```python
from build123d import *

# Parameters (mm, degrees)
BOSS_EXTRUDE1_DEPTH = 48.26
SKETCH2_W           = 9.525
SKETCH2_H           = 22.352
CUT_EXTRUDE1_DEPTH  = 56.99533552
SKETCH3_R           = 1.2192
CUT_EXTRUDE2_DEPTH  = 56.99533552
FILLET2_R           = 1.5875
SKETCH4_R           = 2.5527
CUT_EXTRUDE3_DEPTH  = 56.995335629
CUT_EXTRUDE4_DEPTH  = 56.995335629
CHAMFER2_SIZE       = 6.35
CHAMFER2_SIZE2      = 10.998522628


with BuildPart() as part:
    # Sketch1 → Boss-Extrude1 (new body)
    with BuildSketch(Plane.XY):
        with BuildLine():
            Line((0, 0), (0, -25.4))
            Line((0, -25.4), (1.5875, -25.4))
            ThreePointArc((1.5875, -25.4), (2.710032015, -24.935032015), (3.175, -23.8125))
            Line((3.175, -23.8125), (3.175, -4.7625))
            ThreePointArc((3.175, -4.7625), (3.639967985, -3.639967985), (4.7625, -3.175))
            Line((4.7625, -3.175), (11.1125, -3.175))
            ThreePointArc((11.1125, -3.175), (12.235032015, -2.710032015), (12.7, -1.5875))
            Line((12.7, -1.5875), (12.7, 0))
            Line((12.7, 0), (0, 0))
        make_face()
    extrude(amount=BOSS_EXTRUDE1_DEPTH)

    # Sketch2 → Cut-Extrude1 (cut, through all)
    with BuildSketch(Plane(origin=(0, 0, 0), x_dir=(0, 0, -1), z_dir=(1, 0, 0))):
        with Locations((-4.7625, -14.224)):
            Rectangle(SKETCH2_W, SKETCH2_H)
    extrude(amount=CUT_EXTRUDE1_DEPTH, mode=Mode.SUBTRACT)

    # Sketch3 → Cut-Extrude2 (cut, through all)
    with BuildSketch(Plane(origin=(0, 0, 0), x_dir=(1, 0, 0), z_dir=(0, 1, 0))):
        with Locations(Location((2.794, -3.175, 0), (0, 0, 180))):
            Circle(SKETCH3_R)
        with Locations(Location((7.874, -3.175, 0), (0, 0, 180))):
            Circle(SKETCH3_R)
    extrude(amount=-CUT_EXTRUDE2_DEPTH, mode=Mode.SUBTRACT)

    # Fillet2
    fillet2_edges = [part.edges().sort_by_distance(p)[0] for p in [
        (5.867335197, -3.048, 9.525),
    ]]
    fillet(fillet2_edges, radius=FILLET2_R)

    # Sketch4 → Cut-Extrude3 (cut, through all)
    with BuildSketch(Plane.ZY):
        with Locations(Location((25.4, -9.398, 0), (0, 0, 270))):
            Circle(SKETCH4_R)
    extrude(amount=-CUT_EXTRUDE3_DEPTH, mode=Mode.SUBTRACT)

    # Sketch6 → Cut-Extrude4 (cut, through all)
    with BuildSketch(Plane(origin=(0, 0, 0), x_dir=(1, 0, 0), z_dir=(0, 1, 0))):
        Polygon((5.08, -48.26), (12.7, -1.5875), (12.7, -48.26), align=None)
    extrude(amount=-CUT_EXTRUDE4_DEPTH, mode=Mode.SUBTRACT)

    # Chamfer2
    chamfer2_edges = [part.edges().sort_by_distance(p)[0] for p in [
        (2.54, 0, 48.26),
    ]]
    chamfer2_side = [part.faces().sort_by_distance(p)[0] for p in [
        (1.769133551, -11.790484545, 48.26),
    ]]
    chamfer(chamfer2_edges, length=CHAMFER2_SIZE, length2=CHAMFER2_SIZE2, reference=chamfer2_side[0])


solid = part.part
```
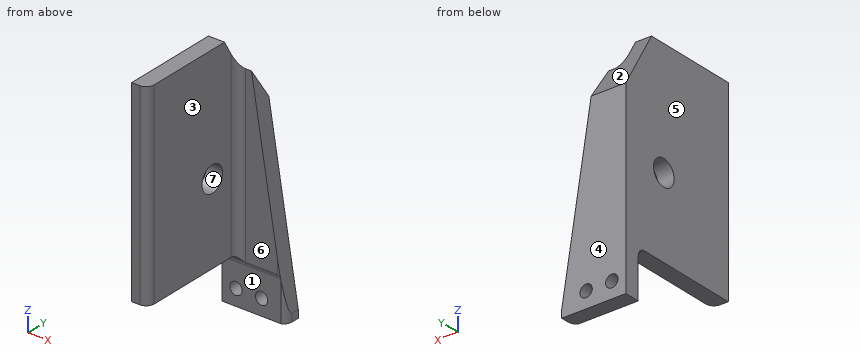
Geometry check sheet. Reference: the model listing, model coordinates, mm. Face numbers are marked on the shaded views. A direction names the side the tool comes from. Give positions to 0.01 mm unless a question says otherwise; leave off trailing zeros. Order: outer loops, then holes, each group sorted by start corner. A loop starts at its lowest first (then second) coordinate and runs counter-clockwise, first axis right, second up.
1. Access from +Z, -Z, +X, -X, +Y, -Y to the whole of each face (thin tool, end or side, straight path). Record for the marked faces 1, 2 and 3.
2. Thickness scan on L1, parallel to X at y = -1.5, z = 4; L2, parallel to X at y = -9, z = 39 (3 decimals); L3, parallel to Y at x = 2.5, z = 25.5. Record the ranges inside material, lowest first.
3. Section check C-C, the plane y = -2.25. Enter the section's corners in (x, z) (3 decimals), and give its area (3 significant figures).
4. Gauge pin test, flat ends, axial feed: pin 1 Ø4 at (y, z) = (-15.5, 30) entering from +X (3 decimals); pin 2 Ø2.5 at (x, z) = (5.5, 2.5) entering from -Y; pin 3 Ø7 at (x, z) = (9, 22.5) entering from -Y (3 decimals). Record the tip position at first contact, or that the pin passes through.
5. Section check D-D, the plane y = -8. Enter the section's corners in (x, z) (3 decimals), and give its area (3 significant figures).
6. Section check B-B, the plane x = 7.75. Enter the section's corners in (y, z) (1 decimal), and give its area (3 significant figures).
7. Section check A-A, the plane z = 27. Enter the section's corners in (x, y) (1 decimal).
8. Release check for a two-part mould opening along Y. For the marked faces 4, 5, 6 and 7 record: pulls with the +Y half, pulls with the -Y half, needs draft (parallel to the pull), parting line crosses it, or undercut.
Values follow:
1. face 1: -Z, +X, -X, -Y
1. face 2: +Z, +X, -X, +Y
1. face 3: +Z, -Z, +X, -Y
2. L1: x = 0 to 1.9, 3.69 to 6.98, 8.77 to 12.31
2. L2: x = 0 to 3.175
2. L3: y = -25.11 to -11.95, -6.85 to 0
3. outline: (0, 0) - (12.555, 0) - (12.555, 2.475) - (6.239, 41.159) - (0, 41.159) - close; hole circle Ø2.438 at (2.794, 3.175); hole circle Ø2.438 at (7.874, 3.175)
3. area: 385 mm2
4. pin 1: stops at x = 3.175
4. pin 2: stops at y = -3.05
4. pin 3: stops at y = -3.175
5. outline: (0, 9.525) - (3.175, 9.525) - (3.175, 23.264) - (0, 23.264) - close; (0, 27.536) - (3.175, 27.536) - (3.175, 48.26) - (0, 48.26) - close
5. area: 109 mm2
6. outline: (-3.2, 8.6) arc R1.6 cw to (-3, 7.9) - (-3, 4.4) - (0, 4.4) - (0, 31.9) - (-3.2, 31.9) - close; (-3, 0) - (0, 0) - (0, 2) - (-3, 2) - close
6. area: 92.8 mm2
7. outline: (0, -25.4) - (1.6, -25.4) arc R1.6 ccw to (3.2, -23.8) - (3.2, -11.4) - (0, -11.4) - close; (0, -7.4) - (3.2, -7.4) - (3.2, -4.8) arc R1.6 cw to (4.8, -3.2) - (8.6, -3.2) - (8.6, 0) - (0, 0) - close
8. face 4: pulls with the +Y half
8. face 5: needs draft
8. face 6: pulls with the -Y half
8. face 7: undercut
